from build123d import *

# Parameters (mm, degrees)
BOSS_EXTRUDE1_DEPTH      = 15
SKETCH2_W                = 5
SKETCH2_H                = 60
BOSS_EXTRUDE2_DEPTH      = 75
CHAMFER1_SIZE            = 30
CHAMFER1_OF_MIRROR1_SIZE = 30
CUT_EXTRUDE3_DEPTH       = 113.472218792
CUT_EXTRUDE4_DEPTH       = 114.688170009
FILLET3_R                = 5
FILLET4_R                = 2
CUT_EXTRUDE6_DEPTH       = 106.475115549
CUT_EXTRUDE6_DEPTH_BACK  = 106.475115549
SKETCH8_R                = 2.5


# Some blends are built 0.0001 mm under size
with BuildPart() as part:
    # Sketch1 → Boss-Extrude1 (new, symmetric)
    with BuildSketch(Plane(origin=(0, 0, 0), x_dir=(0, 0, -1), z_dir=(1, 0, 0))):
        Polygon((20, 10), (-20, 10), (-20, -10), (20, -10), (20, -15), (-25, -15), (-25, 15), (20, 15), align=None)
    extrude(amount=BOSS_EXTRUDE1_DEPTH, both=True)

    # Sketch2 → Boss-Extrude2 (add)
    with BuildSketch(Plane.XY.offset(25)):
        with Locations((-12.5, 15)):
            Rectangle(SKETCH2_W, SKETCH2_H)
    boss_extrude2 = extrude(amount=BOSS_EXTRUDE2_DEPTH)

    # Chamfer1
    chamfer1_edges = [part.edges().sort_by_distance(p)[0] for p in [
        (-12.5, 45, 25),
    ]]
    chamfer(chamfer1_edges, length=CHAMFER1_SIZE - 0.0001)  # a hair under: the kernel refuses the full size

    # Mirror1: Boss-Extrude2 across plane
    add(boss_extrude2.mirror(Plane(origin=(0, 0, 0), x_dir=(0, 0, 1), z_dir=(1, 0, 0))))

    # Chamfer1 of Mirror1
    chamfer1_of_mirror1_edges = [part.edges().sort_by_distance(p)[0] for p in [
        (12.5, 45, 25),
    ]]
    chamfer(chamfer1_of_mirror1_edges, length=CHAMFER1_OF_MIRROR1_SIZE - 0.0001)  # a hair under: the kernel refuses the full size

    # Sketch5 → Cut-Extrude3 (cut, through all)
    with BuildSketch(Plane(origin=(-10, 0, 0), x_dir=(0, 0, -1), z_dir=(1, 0, 0))):
        Polygon((-25, -15), (-25, 15), (-55, 45), (-100, 45), (-100, -15), align=None)
    extrude(amount=-CUT_EXTRUDE3_DEPTH, mode=Mode.SUBTRACT)

    # Sketch6 → Cut-Extrude4 (cut, through all)
    with BuildSketch(Plane(origin=(15, 0, 0), x_dir=(0, 0, -1), z_dir=(1, 0, 0))):
        with BuildLine():
            Line((-62.5, 0), (-72.5, 0))
            ThreePointArc((-72.5, 0), (-87.5, 15), (-72.5, 30))
            Line((-72.5, 30), (-62.5, 30))
            ThreePointArc((-62.5, 30), (-47.5, 15), (-62.5, 0))
        make_face()
    extrude(amount=-CUT_EXTRUDE4_DEPTH, mode=Mode.SUBTRACT)

    # Fillet3
    # the kernel refuses this fillet: 5 mm, written as the material it adds along each edge
    with BuildSketch(Plane(origin=(10, 27.5, 25), x_dir=(0, 0, 1), z_dir=(0, -1, 0))) as fillet3_piece_1_section:
        with BuildLine():
            CenterArc((FILLET3_R, FILLET3_R), FILLET3_R, 180, 90)
            Line((0, FILLET3_R), (0, 0))
            Line((0, 0), (FILLET3_R, 0))
        make_face()
    fillet3_piece_1 = extrude(amount=42.5, mode=Mode.PRIVATE)
    fillet3_piece_1 = split(fillet3_piece_1, bisect_by=Plane(origin=(9.467598147, 16.61296207, 26.61286207), z_dir=(0, -0.7071067811865476, 0.7071067811865476)), keep=Keep.TOP, mode=Mode.PRIVATE)
    fillet3_piece_1 = split(fillet3_piece_1, bisect_by=Plane(origin=(9.467598147, 15, 27.150516093), z_dir=(0, 1, 0)), keep=Keep.TOP, mode=Mode.PRIVATE)
    add(fillet3_piece_1)
    with BuildSketch(Plane(origin=(10, 15, 25), x_dir=(0, 0, 1), z_dir=(0, -1, 0))) as fillet3_piece_2_section:
        with BuildLine():
            CenterArc((FILLET3_R, FILLET3_R), FILLET3_R, 180, 90)
            Line((0, FILLET3_R), (0, 0))
            Line((0, 0), (FILLET3_R, 0))
        make_face()
    fillet3_piece_2 = extrude(amount=30, mode=Mode.PRIVATE)
    fillet3_piece_2 = split(fillet3_piece_2, bisect_by=Plane(origin=(8.982634351, 0, 25), z_dir=(0, 0, 1)), keep=Keep.TOP, mode=Mode.PRIVATE)
    add(fillet3_piece_2)

    # Fillet4
    fillet4_edges = [part.edges().sort_by_distance(p)[0] for p in [
        (-15, 0, 25),
    ]]
    fillet(fillet4_edges, radius=FILLET4_R)

    # Sketch8 → Cut-Extrude6 (cut, two sides: drawn at the far end of the back side and taken through both)
    with BuildSketch(Plane(origin=(0, 15, 0), x_dir=(1, 0, 0), z_dir=(0, 1, 0)).offset(-CUT_EXTRUDE6_DEPTH_BACK)):
        with Locations(Location((-7.5, -10, 0), (0, 0, 270))):
            Circle(SKETCH8_R)
        with Locations(Location((7.5, -10, 0), (0, 0, 270))):
            Circle(SKETCH8_R)
        with Locations(Location((-7.5, 10, 0), (0, 0, 270))):
            Circle(SKETCH8_R)
        with Locations(Location((7.5, 10, 0), (0, 0, 270))):
            Circle(SKETCH8_R)
    extrude(amount=CUT_EXTRUDE6_DEPTH + CUT_EXTRUDE6_DEPTH_BACK, mode=Mode.SUBTRACT)


solid = part.part
Design review of the part built by this model. Coordinates are the model's own, in mm. A direction names the side the tool comes from. Give positions to 0.01 mm unless a question says otherwise; leave off trailing zeros. Loops run counter-clockwise (first coordinate to the right, second up) from the corner with the lowest first, then second, coordinate; pieces in that order, holes last. Notation, with made-up numbers: M 69,-35.75 L 75,-35.75 A18 ccw 75,-8.75 Z; hole C -23,78.25 d3. An arc over 180 degrees is marked long. One line per question, with ' | ' between items. Start each with the question number.
1. Insertion check: P1, Ø8, axis at x = -7.5, z = 10, coming from the +Y side; P2, Ø4, axis at x = 11.5, y = 7, coming from the -Z side; P3, Ø18, axis at y = 11, z = 73.5, coming from the -X side; P4, Ø14.5, axis at x = -3, y = 1.5, coming from the +Z side. Each pin has a flat end and moves straight along its axis. Give the tip position at first contact, or say it passes through.
2. Add section B-B (z = 64). Write out the cut boundary in (x, y).
3. To check wall thickness, follow L1, parallel to X at y = 13.2, z = 10; L2, parallel to Y at x = 12.75, z = -11.5; L3, parallel to Z at x = 7.5, y = -13.55. State the ranges of each line that lie inside material, in increasing order.
4. For faces 5 (the face through (0, 13, -20)), 6 (the face through (0, 10, 0)), 7 (the face through (13, 45, 77)), 8 (the face through (12.535, 14.67, 87.496)), 9 (the face through (0, 15, 3)), list the 3-axis set-ups (+Z, -Z, +X, -X, +Y, -Y) from which the entire face can be reached by the end or side of a thin tool; tool diameter is ignored.
5. Add section A-A (x = -7.5). Write out the cut boundary in (y, z), plus the area to 3 significant figures.
6. The part is to be moulded in two halves that separate along X. For faces 1 (the face through (0, 0, 20)), 2 (the face through (-15, -10.2, 6)), 3 (the face through (5.06, 12.47, 9.46)), 4 (the face through (-9.94, -12.53, 9.46)), say which applies: released by +X, released by -X, zero draft, split by the parting line, or undercut.
7. Add section D-D (z = 49). Write out the cut boundary in (x, y), plus the area to 3 significant figures.
Worked out:
1) P1: stops at y = 15 | P2: stops at z = 20 | P3: passes through | P4: stops at z = 25
2) outline: M 10,-15 L 15,-15 L 15,0 L 10,0 Z; M 10,30 L 15,30 L 15,45 L 10,45 Z
3) L1: x = -15 to -10, -5 to 5, 10 to 15 | L2: y = -15 to -10, 10 to 15 | L3: z = -20 to -12.5, -7.5 to 7.5, 12.5 to 25.67
4) face 5: -Z, +X, -X, +Y, -Y | face 6: -Z, +X, -X | face 7: +Z, -Z, +X, -X, +Y | face 8: +X, -X | face 9: -Z, +X, -X, +Y
5) outline: M -15,-20 L -10,-20 L -10,-12.5 L -15,-12.5 Z; M -15,-7.5 L -10,-7.5 L -10,7.5 L -15,7.5 Z; M -15,12.5 L -10,12.5 L -10,20 L 10,20 L 10,12.5 L 15,12.5 L 15,25 L -15,25 Z; M 10,-20 L 15,-20 L 15,-12.5 L 10,-12.5 Z; M 10,-7.5 L 15,-7.5 L 15,7.5 L 10,7.5 Z | area: 450 mm²
6) face 1: zero draft | face 2: released by -X | face 3: undercut | face 4: undercut
7) outline: M 10,-15 L 15,-15 L 15,8.46 L 10,8.46 Z; M 10,21.54 L 15,21.54 L 15,39 L 10,39 Z | area: 205 mm²
